Input: part model. Units: mm. Frame: model coordinates. Face numbers are marked on the shaded views. A direction names the side the tool comes from. Coordinates: 2 decimals unless noted, no trailing zeros. Loops run counter-clockwise (first coordinate to the right, second up) from the corner with the lowest first, then second, coordinate; pieces in that order, holes last.
Item 1: Pull-direction query (X, two-part tool) for the marked faces 3, 4 and 5; classes: released by +X, released by -X, zero draft, split by the parting line, or undercut.
Item 2: Section A-A on z = 10. Return loops of the section in (x, y), and give its area (3 significant figures).
Item 3: Contact query for flat-ended pins moving along their axis: P1, Ø5, axis at y = 30, z = -104, coming from the +X side; P2, Ø6, axis at y = 29, z = -91, coming from the +X side; P3, Ø10, axis at x = -6.5, y = 13, coming from the +Z side; P4, Ø12, axis at y = 7, z = -11.5, coming from the +X side. Output: stop coordinate, or through.
Item 4: Ray query, line 1 along Y through (x, z) = (0, 2.15); line 2 along Y through (x, z) = (45.5, -6); line 3 along Z through (x, y) = (-19, 37). Return the intervals inside material, ascending.
Item 5: Reachability of the marked faces 1 and 2 from +Z, -Z, +X, -X, +Y, -Y: full face, straight path, thin tool, end or side. Return the list, or none.
Item 6: Section B-B on z = -137. Return loops of the section in (x, y).
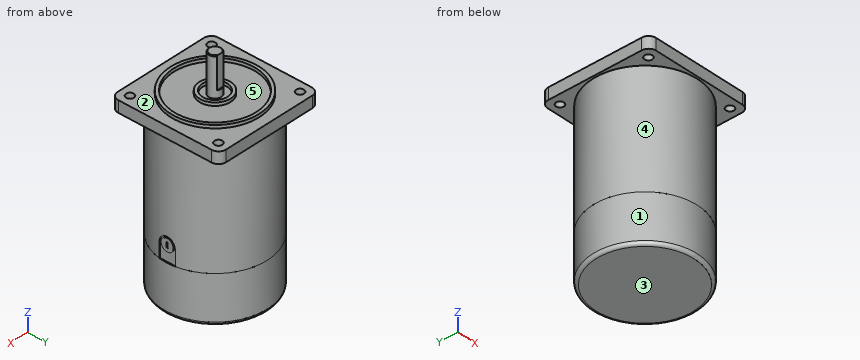
```python
from build123d import *

# Parameters (mm, degrees)
SKETCH_3_W               = 104
SKETCH_3_H               = 104
EXTRUDE_1_DEPTH          = 11
SKETCH_4_R               = 3.75
CUT_EXTRUDE_1_DEPTH      = 11
PATTERN_CIRCULAR_1_COUNT = 4
FILLET_1_R               = 7.2
SKETCH_5_W               = 6.63324958
SKETCH_5_H               = 1
CUT_EXTRUDE_2_DEPTH      = 30
FILLET_2_R               = 3
CUT_EXTRUDE_START        = 50
CUT_EXTRUDE_3_DEPTH      = 1
SKETCH_7_R               = 6
EXTRUDE_2_DEPTH          = 0.5
CHAMFER_2_SIZE           = 0.62
MOVE_BODY_1_ANGLE        = 90


with BuildPart() as part:
    # 草图2 → 旋转1 (revolve)
    with BuildSketch(Plane.XY, mode=Mode.PRIVATE) as revolve_1_sk:
        Polygon((0, 15), (-3, 15), (-3, 12), (0, 12), (0, 6), (-37, 6), (-37, 0), (165, 0), (165, 50), (120, 50), (120, 42.5), (119.99, 42.5), (119.99, 50), (0, 50), (0, 42.5), (-3, 42.5), (-3, 39.5), (0, 39.5), align=None)
    revolve(revolve_1_sk.sketch.rotate(Axis((-37, 0, 0), (1, 0, 0)), 90), axis=Axis((-37, 0, 0), (1, 0, 0)))

    # 草图3 → 凸台-拉伸1 (add)
    with BuildSketch(Plane.ZY):
        Rectangle(SKETCH_3_W, SKETCH_3_H)
    extrude(amount=-EXTRUDE_1_DEPTH)

    # 草图4 → 切除-拉伸1 (cut)
    with BuildSketch(Plane.ZY):
        with Locations((42.426406871, 42.426406871)):
            Circle(SKETCH_4_R)
    cut_extrude_1 = extrude(amount=-CUT_EXTRUDE_1_DEPTH, mode=Mode.SUBTRACT)

    # 阵列(圆周)1: 切除-拉伸1 ×4 about axis
    pattern_circular_1_axis = Axis((0, 0, 0), (1, 0, 0))
    for i in range(1, PATTERN_CIRCULAR_1_COUNT):
        add(cut_extrude_1.rotate(pattern_circular_1_axis, i * 360 / PATTERN_CIRCULAR_1_COUNT), mode=Mode.SUBTRACT)

    # 圆角1
    fillet_1_edges = [part.edges().sort_by_distance(p)[0] for p in [
        (5.5, -52, -52),
        (5.5, 52, -52),
        (5.5, 52, 52),
        (5.5, -52, 52),
    ]]
    fillet(fillet_1_edges, radius=FILLET_1_R)

    # 草图5 → 切除-拉伸2 (cut)
    with BuildSketch(Plane.ZY.offset(37)):
        with Locations((0, 5.5)):
            Rectangle(SKETCH_5_W, SKETCH_5_H)
    extrude(amount=-CUT_EXTRUDE_2_DEPTH, mode=Mode.SUBTRACT)

    # 圆角2
    fillet_2_edges = [part.edges().sort_by_distance(p)[0] for p in [
        (165, 0, -50),
    ]]
    fillet(fillet_2_edges, radius=FILLET_2_R)

    # 草图6 → 切除-拉伸3 (cut)
    with BuildSketch(Plane.XY.offset(CUT_EXTRUDE_START)):
        with BuildLine():
            Line((105, 7.5), (120, 7.5))
            Line((120, 7.5), (120, -7.5))
            Line((120, -7.5), (105, -7.5))
            ThreePointArc((105, -7.5), (97.5, 0), (105, 7.5))
        make_face()
    extrude(amount=-CUT_EXTRUDE_3_DEPTH, mode=Mode.SUBTRACT)

    # 草图7 → 凸台-拉伸2 (add)
    with BuildSketch(Plane.XY.offset(49)):
        with Locations((105, 0)):
            Circle(SKETCH_7_R)
        with BuildLine():
            Line((103, 0.75), (107, 0.75))
            ThreePointArc((107, 0.75), (107.75, 0), (107, -0.75))
            Line((107, -0.75), (103, -0.75))
            ThreePointArc((103, -0.75), (102.25, 0), (103, 0.75))
        make_face(mode=Mode.SUBTRACT)
    extrude(amount=EXTRUDE_2_DEPTH)

    # 倒角2
    chamfer_2_edges = [part.edges().sort_by_distance(p)[0] for p in [
        (-37, -5.286764074, -2.837274331),
    ]]
    chamfer(chamfer_2_edges, length=CHAMFER_2_SIZE)


with BuildPart() as part_1:
    # Move Body 1: moved
    add(part.part.rotate(Axis((0, 0, 0), (0, 1, 0)), MOVE_BODY_1_ANGLE))


solid = part_1.part
```
Results found:
1. face 3: zero draft
1. face 4: split by the parting line
1. face 5: undercut
2. outline: (-3.32, 5) arc R6 ccw (long way) to (3.32, 5) - close
2. area: 109 mm2
3. P1: stops at x = 41.76
3. P2: stops at x = 42.71
3. P3: stops at z = 3
3. P4: stops at x = 52
4. line 1: y = -42.5 to -39.5, -15 to -12, -6 to 6, 12 to 15, 39.5 to 42.5
4. line 2: y = -51.97 to -44.57, -40.28 to 40.28, 44.57 to 51.97
4. line 3: z = -165 to 3
5. face 1: -Z
5. face 2: +Z
6. outline: circle Ø100 at (0, 0)
